```python
from build123d import *

# Parameters (mm, degrees)
F0_W     = 80
F0_H     = 100
F1_DEPTH = 20
F1_TAPER = 2
F2_W     = 60
F2_H     = 80
F3_DEPTH = 7
F3_TAPER = -1
F4_R     = 1
F5_R     = 0.6


with BuildPart() as f1:
    # F0 (on Top) → F1 (new body)
    with BuildSketch(Plane.XY):
        Rectangle(F0_W, F0_H)
    extrude(amount=F1_DEPTH, taper=F1_TAPER)

    # F2 (on face) → F3 (join)
    with BuildSketch(Plane.XY.offset(20)):
        Rectangle(F2_W, F2_H)
    extrude(amount=F3_DEPTH, taper=F3_TAPER)

    # F4
    f4_edges = [f1.edges().sort_by_distance(p)[0] for p in [
        (-39.650792, 49.650792, 10),
        (39.650792, 49.650792, 10),
        (39.650792, -49.650792, 10),
        (-39.650792, -49.650792, 10),
        (0, 49.301585, 20),
        (-39.301585, 0, 20),
        (0, -49.301585, 20),
        (39.301585, 0, 20),
    ]]
    fillet(f4_edges, radius=F4_R)

    # F5
    f5_edges = [f1.edges().sort_by_distance(p)[0] for p in [
        (-30.061093, 40.061093, 23.5),
        (-30.122185, 0, 27),
        (0, 40.122185, 27),
        (30.061093, 40.061093, 23.5),
        (30.122185, 0, 27),
        (30.061093, -40.061093, 23.5),
        (0, -40.122185, 27),
        (-30.061093, -40.061093, 23.5),
    ]]
    fillet(f5_edges, radius=F5_R)


solid = f1.part
```
Verification items for the finished model (mm, model axes). Coordinates: 2 decimals unless noted, no trailing zeros. Loops run counter-clockwise (first coordinate to the right, second up) from the corner with the lowest first, then second, coordinate; pieces in that order, holes last. Notation, with made-up numbers: (74, 78.5) - (118, 78.5) arc R12 ccw to (118, 99.5) - close; hole circle Ø3 at (-36, -10.5). An arc over 180 degrees is marked (long way). Answer as a JSON object with one key per item and string values.
(1) Scan lines: line 1 along X through (y, z) = (-13, 14.75); line 2 along Y through (x, z) = (-1, 18.5); line 3 along Z through (x, y) = (34.5, 2). Record each from-to range of solid material in increasing order.
Response:
{"line 1": "x = -39.48 to 39.48", "line 2": "y = -49.35 to 49.35", "line 3": "z = 0 to 20"}
(2) Go/stop test with flat-tipped pins: pin 1 Ø5 at (y, z) = (-4.5, 22) entering from -X; pin 2 Ø6 at (y, z) = (3.5, 5.5) entering from +X; pin 3 Ø12 at (x, z) = (-28.5, 7) entering from +Y. Record where each tip stops, or that it passes through.
Response:
{"pin 1": "stops at x = -39.2", "pin 2": "stops at x = 39.91", "pin 3": "stops at y = 49.97"}
(3) Cross-section at A-A, the plane x = 34. Record the boundary of the cut face in (y, z).
Response:
{"outline": "(-50, 0) - (50, 0) - (49.34, 19.03) arc R1 ccw to (48.34, 20) - (-48.34, 20) arc R1 ccw to (-49.34, 19.03) - close"}
